The listing builds one solid part. Answer for the finished solid, in the listing's coordinates (mm). A direction names the side the tool comes from. Give positions to 0.01 mm unless a question says otherwise; leave off trailing zeros. Loops run counter-clockwise (first coordinate to the right, second up) from the corner with the lowest first, then second, coordinate; pieces in that order, holes last.
Item 1: Each of these flat-tipped pins is pushed along its axis until it touches: pin 1 Ø6.5 at (x, y) = (-3, -9.5) entering from +Z; pin 2 Ø5 at (x, z) = (-3, 28) entering from +Y; pin 3 Ø4 at (x, y) = (-9.5, 2) entering from +Z. Where does it stop, or does it pass through?
Item 2: Section D-D, the plane x = -3.25 is taken. Give the vertices of the cut face in (y, z), and give its area (3 significant figures).
Item 3: Consider line 1 along Y through (x, z) = (0, 0.75); line 2 along Z through (x, y) = (0, 3.8); line 3 along Z through (x, y) = (9, 6). Determine where each line is inside the solid, lowest interval first.
Item 4: A tool of negligible diameter and unlimited length cuts with its end or side. For faces 4 (the face through (-6.5, 0, 2)), 5 (the face through (6.5, 0, 2)), 6 (the face through (0, 6.5, 27)), 7 (the face through (8.389, 4.355, 33.147)), from which of +Z, -Z, +X, -X, +Y, -Y can it reach the whole face along a straight path? Write none if from no direction.
Item 5: The mould has two halves that part along X. Classify faces 1 (the face through (0.091, 6.856, 3.676)), 2 (the face through (-6.58, 4.36, 42.3)), 3 (the face through (7.98, 4.36, 13.12)): pulls with the +X half, pulls with the -X half, needs draft (parallel to the pull), parting line crosses it, or undercut.
Item 6: Section C-C, the plane x = 8.25 is taken. Give the vertices of the cut face in (y, z), and give its area (3 significant figures).
Item 7: Section A-A, the plane x = 0 is taken. Give the number of separate pieces and of enclosed holes in the cut face, and give its area (3 significant figures).
Item 8: Section B-B, the plane y = 10 is taken. Give the vertices of the cut face in (x, z).
from build123d import *

# Parameters (mm, degrees)
ESQUISSE1_W             = 13
ESQUISSE1_H             = 30
ESQUISSE1_R             = 1.65
BOSS_EXTRU_1_DEPTH      = 3.3
CONG_1_R                = 2
ESQUISSE2_W             = 13
ESQUISSE2_H             = 4.34999702
BOSS_EXTRU_2_DEPTH      = 2.77
ESQUISSE4_R             = 6.8
BOSS_EXTRU_4_DEPTH      = 4.349997
ESQUISSE6_R             = 1.15
ENL_V_MAT_EXTRU_2_DEPTH = 22.49999702
ESQUISSE8_R             = 2
ESQUISSE8_R_2           = 1.25
BOSS_EXTRU_5_DEPTH      = 4.349997
CONG_2_R                = 1.25


with BuildPart() as part:
    # Esquisse1 → Boss.-Extru.1 (new body)
    with BuildSketch(Plane.XY):
        Rectangle(ESQUISSE1_W, ESQUISSE1_H)
        with Locations((0, 10)):
            Circle(ESQUISSE1_R, mode=Mode.SUBTRACT)
        with Locations((0, -10)):
            Circle(ESQUISSE1_R, mode=Mode.SUBTRACT)
    extrude(amount=BOSS_EXTRU_1_DEPTH)

    # Congé1
    cong_1_edges = [part.edges().sort_by_distance(p)[0] for p in [
        (6.5, -15, 1.65),
        (-6.5, -15, 1.65),
        (-6.5, 15, 1.65),
        (6.5, 15, 1.65),
    ]]
    fillet(cong_1_edges, radius=CONG_1_R)

    # Esquisse2 → Boss.-Extru.2 (add)
    with BuildSketch(Plane.XY.offset(3.3)):
        with Locations((0, 4.32499851)):
            Rectangle(ESQUISSE2_W, ESQUISSE2_H)
    extrude(amount=BOSS_EXTRU_2_DEPTH)

    # Esquisse4 → Boss.-Extru.4 (add)
    with BuildSketch(Plane(origin=(0, 6.49999702, 0), x_dir=(1, 0, 0), z_dir=(0, 1, 0))):
        with BuildLine():
            Line((-6.5, -6.07), (6.5, -6.07))
            ThreePointArc((6.5, -6.07), (12.5, -16.747078252), (6.5, -27.424156504))
            Line((6.5, -27.424156504), (-6.5, -27.424156504))
            ThreePointArc((-6.5, -27.424156504), (-12.5, -16.747078252), (-6.5, -6.07))
        make_face()
        with Locations((0, -16.747078252)):
            Circle(ESQUISSE4_R, mode=Mode.SUBTRACT)
    extrude(amount=-BOSS_EXTRU_4_DEPTH)

    # Esquisse6 → Enlèv. mat.-Extru.2 (cut, through all)
    with BuildSketch(Plane(origin=(0, 6.49999702, 0), x_dir=(1, 0, 0), z_dir=(0, 1, 0))):
        with Locations((0, -7.247078252)):
            Circle(ESQUISSE6_R)
        with Locations((-8.227241336, -11.997078252)):
            Circle(ESQUISSE6_R)
        with Locations((8.227241336, -11.997078252)):
            Circle(ESQUISSE6_R)
        with Locations((-8.227241336, -21.497078252)):
            Circle(ESQUISSE6_R)
        with Locations((8.227241336, -21.497078252)):
            Circle(ESQUISSE6_R)
    extrude(amount=-ENL_V_MAT_EXTRU_2_DEPTH, mode=Mode.SUBTRACT)

    # Esquisse8 → Boss.-Extru.5 (add)
    with BuildSketch(Plane(origin=(0, 6.49999702, 0), x_dir=(1, 0, 0), z_dir=(0, 1, 0))):
        with BuildLine():
            Line((0, -51.937078252), (-12.5, -33.625808063))
            Line((-12.5, -33.625808063), (-12.5, -16.747078252))
            ThreePointArc((-12.5, -16.747078252), (-10.897247359, -22.870802609), (-6.5, -27.424156504))
            Line((-6.5, -27.424156504), (6.5, -27.424156504))
            ThreePointArc((6.5, -27.424156504), (10.897247359, -22.870802609), (12.5, -16.747078252))
            Line((12.5, -16.747078252), (12.5, -33.627078252))
            Line((12.5, -33.627078252), (0, -51.937078252))
        make_face()
        with Locations((0, -36.927078252)):
            Circle(ESQUISSE8_R, mode=Mode.SUBTRACT)
        with Locations((8.660254038, -31.927078252)):
            Circle(ESQUISSE8_R_2, mode=Mode.SUBTRACT)
        with Locations((-8.660254038, -31.927078252)):
            Circle(ESQUISSE8_R_2, mode=Mode.SUBTRACT)
        with Locations((0, -46.937078252)):
            Circle(ESQUISSE8_R_2, mode=Mode.SUBTRACT)
    extrude(amount=-BOSS_EXTRU_5_DEPTH)

    # Congé2
    cong_2_edges = [part.edges().sort_by_distance(p)[0] for p in [
        (-12.5, 4.32499852, 33.625808063),
        (0, 4.32499852, 51.937078252),
        (12.5, 4.32499852, 33.627078252),
        (0, 6.49999702, 3.3),
        (0, 2.15, 3.3),
        (6.5, 4.32499851, 6.07),
        (-6.5, 4.32499851, 6.07),
    ]]
    fillet(cong_2_edges, radius=CONG_2_R)


solid = part.part
Worked answers:
1. pin 1: stops at z = 3.3
1. pin 2: stops at y = 6.5
1. pin 3: stops at z = 40.94
2. outline: (-15, 0) - (15, 0) - (15, 3.3) - (7.75, 3.3) arc R1.25 cw to (6.5, 4.55) - (6.5, 10.77) - (2.15, 10.77) - (2.15, 4.55) arc R1.25 cw to (0.9, 3.3) - (-15, 3.3) - close; (2.15, 22.72) - (6.5, 22.72) - (6.5, 47.18) - (2.15, 47.18) - close
2. area: 239 mm2
3. line 1: y = -15 to -11.65, -8.35 to 8.35, 11.65 to 15
3. line 2: z = 0 to 6.1, 8.4 to 9.95, 23.55 to 34.93, 38.93 to 45.69, 48.19 to 50.97
3. line 3: z = 8.07 to 11.15, 12.85 to 20.65, 22.35 to 30.72, 33.13 to 38.75
4. face 4: -Z, -X, +Y, -Y
4. face 5: -Z, +X, +Y, -Y
4. face 6: +Z, +X, -X, +Y
4. face 7: +Y, -Y
5. face 1: needs draft
5. face 2: pulls with the -X half
5. face 3: undercut
6. outline: (2.15, 7.36) - (6.5, 7.36) - (6.5, 10.85) - (2.15, 10.85) - close; (2.15, 13.15) - (6.5, 13.15) - (6.5, 20.35) - (2.15, 20.35) - close; (2.15, 22.65) - (6.5, 22.65) - (6.5, 30.75) - (2.15, 30.75) - close; (2.15, 33.11) - (6.5, 33.11) - (6.5, 39.85) - (2.15, 39.85) - close
6. area: 111 mm2
7. separate pieces: 7
7. enclosed holes: 0
7. area: 188 mm2
8. outline: (-6.5, 0) - (-1.65, 0) - (-1.65, 3.3) - (-6.5, 3.3) - close; (1.65, 0) - (6.5, 0) - (6.5, 3.3) - (1.65, 3.3) - close
